Model file for the job. Use its own axes, mm. Face numbers are marked on the shaded views. A direction names the side the tool comes from. Coordinates: 2 decimals unless noted, no trailing zeros. Write each loop counter-clockwise with the first axis right and the second up, starting at its lowest first coordinate (ties: lowest second). Pieces come first, ordered by that corner, then holes.
Q1. Which spindle directions (+Z, -Z, +X, -X, +Y, -Y) get a long thin tool onto all of the face, cutting with end or side? Do the marked faces 1, 2 and 3. Say none if no direction does.
Q2. Drill centre lines: probe 1 along Y at (x, z) = (3.75, -9); probe 2 along X at (y, z) = (17.25, 0); probe 3 along Z at (x, y) = (-11.25, 7). Where is each one in solid material? Low to high.
Q3. Band-saw the part on C-C, the plane z = 1. State how many separate pieces and enclosed holes the cut face has, plus the area to 3 significant figures.
Q4. Band-saw the part on B-B, the plane x = -1.5. Write the cut outline in (y, z).
Q5. Band-saw the part on D-D, the plane y = 9. Write the cut outline in (x, z), plus the area to 3 significant figures.
Q6. Pin check, flat tips, straight feed: P1, Ø5.5, axis at y = 5, z = 1, coming from the -X side; P2, Ø10, axis at x = -4, z = -4, coming from the -Y side; P3, Ø12, axis at x = 1.5, z = -2, coming from the -Y side; P4, Ø3, axis at y = 13.5, z = 6.5, coming from the +X side. Stop position of each tip, or through.
Q7. Pull direction Z, two halves, no side cores. Call the marked faces 4, 5 and 6: released by +Z, released by -Z, zero draft, split by the parting line, or undercut.
Q8. Band-saw the part on A-A, the plane y = 39. Write the cut outline in (x, z), plus the area to 3 significant figures.
from build123d import *

# Parameters (mm, degrees)
SKETCH1_R               = 12.7
BOSS_EXTRUDE1_DEPTH     = 45.3136
CUT_EXTRUDE1_START      = -11.43
CUT_EXTRUDE1_DEPTH      = 11.43
CUT_EXTRUDE2_DEPTH      = 11.43
CUT_EXTRUDE3_DEPTH      = 52.259289353
CUT_EXTRUDE3_DEPTH_BACK = 52.259289353
SKETCH4_R               = 3.175
SKETCH5_R               = 2.54
CUT_EXTRUDE4_DEPTH      = 39.349424517
BOSS_EXTRUDE2_REACH     = 53.259
BOSS_EXTRUDE3_DEPTH     = 1.27


with BuildPart() as part:
    # Sketch1 → Boss-Extrude1 (new body)
    with BuildSketch(Plane(origin=(0, 0, 0), x_dir=(1, 0, 0), z_dir=(0, 1, 0))):
        with Locations(Location((0, 0, 0), (0, 0, 90))):
            Circle(SKETCH1_R)
    extrude(amount=BOSS_EXTRUDE1_DEPTH)

    # Sketch2 → Cut-Extrude1 (cut)
    with BuildSketch(Plane(origin=(0, 45.3136, 0), x_dir=(1, 0, 0), z_dir=(0, 1, 0)).offset(CUT_EXTRUDE1_START)):
        with BuildLine():
            Line((7.62, 10.16), (7.62, -10.16))
            ThreePointArc((7.62, -10.16), (0, -12.7), (-7.62, -10.16))
            Line((-7.62, -10.16), (-7.62, 10.16))
            ThreePointArc((-7.62, 10.16), (0, 12.7), (7.62, 10.16))
        make_face()
    extrude(amount=CUT_EXTRUDE1_DEPTH, mode=Mode.SUBTRACT)

    # Sketch3 → Cut-Extrude2 (cut)
    with BuildSketch(Plane.XZ):
        with BuildLine():
            Line((-7.62, 10.16), (-7.62, -10.16))
            ThreePointArc((-7.62, -10.16), (0, -12.7), (7.62, -10.16))
            Line((7.62, -10.16), (7.62, 10.16))
            ThreePointArc((7.62, 10.16), (0, 12.7), (-7.62, 10.16))
        make_face()
    extrude(amount=-CUT_EXTRUDE2_DEPTH, mode=Mode.SUBTRACT)

    # Sketch4 → Cut-Extrude3 (cut, two sides: drawn at the far end of the back side and taken through both)
    with BuildSketch(Plane(origin=(-7.62, 0, 0), x_dir=(0, 0, -1), z_dir=(1, 0, 0)).offset(-CUT_EXTRUDE3_DEPTH_BACK)):
        with Locations(Location((0, 40.2336, 0), (0, 0, 270))):
            Circle(SKETCH4_R)
        with Locations(Location((0, 5.08, 0), (0, 0, 270))):
            Circle(SKETCH4_R)
        with BuildLine():
            Line((0, 45.3136), (-10.16, 45.3136))
            Line((-10.16, 45.3136), (-10.16, 33.8836))
            Line((-10.16, 33.8836), (-4.264917923, 42.993468677))
            ThreePointArc((-4.264917923, 42.993468677), (-2.427577715, 44.696028312), (0, 45.3136))
        make_face()
        with BuildLine():
            Line((-10.16, 11.43), (-10.16, 0))
            Line((-10.16, 0), (0, 0))
            ThreePointArc((0, 0), (-2.427577715, 0.617571688), (-4.264917923, 2.320131323))
            Line((-4.264917923, 2.320131323), (-10.16, 11.43))
        make_face()
    extrude(amount=CUT_EXTRUDE3_DEPTH + CUT_EXTRUDE3_DEPTH_BACK, mode=Mode.SUBTRACT)

    # Sketch5 → Cut-Extrude4 (cut, through all)
    with BuildSketch(Plane(origin=(0, 33.8836, 0), x_dir=(1, 0, 0), z_dir=(0, 1, 0))):
        with Locations(Location((0, 0, 0), (0, 0, 270))):
            Circle(SKETCH5_R)
    extrude(amount=-CUT_EXTRUDE4_DEPTH, mode=Mode.SUBTRACT)

    # Boss-Extrude2: up to this face of the body (flat: up to its plane)
    boss_extrude2_end = Plane(part.part.faces().sort_by_distance((7.62, 34.116741009, 0))[0])
    # Sketch6 → Boss-Extrude2 (add, up to the picked face)
    with BuildSketch(Plane(origin=(-7.62, 0, 0), x_dir=(0, 0, -1), z_dir=(1, 0, 0)), mode=Mode.PRIVATE) as boss_extrude2_sk1:
        Polygon((2.54, 33.8836), (10.16, 33.8836), (10.16, 35.1536), (7.62, 35.1536), align=None)
    boss_extrude2_tool1 = split(extrude(boss_extrude2_sk1.sketch, amount=BOSS_EXTRUDE2_REACH, mode=Mode.PRIVATE), bisect_by=boss_extrude2_end, keep=Keep.BOTH, mode=Mode.PRIVATE)
    add(boss_extrude2_tool1.solids().sort_by(Axis((-7.62, 34.412767, -7.408333), (1, 0, 0)))[0])

    # Sketch7 → Boss-Extrude3 (add)
    with BuildSketch(Plane(origin=(0, 33.8836, 0), x_dir=(1, 0, 0), z_dir=(0, 1, 0))):
        with BuildLine():
            Line((-7.62, 10.16), (7.62, 10.16))
            ThreePointArc((7.62, 10.16), (0, 12.7), (-7.62, 10.16))
        make_face()
    extrude(amount=BOSS_EXTRUDE3_DEPTH)


solid = part.part
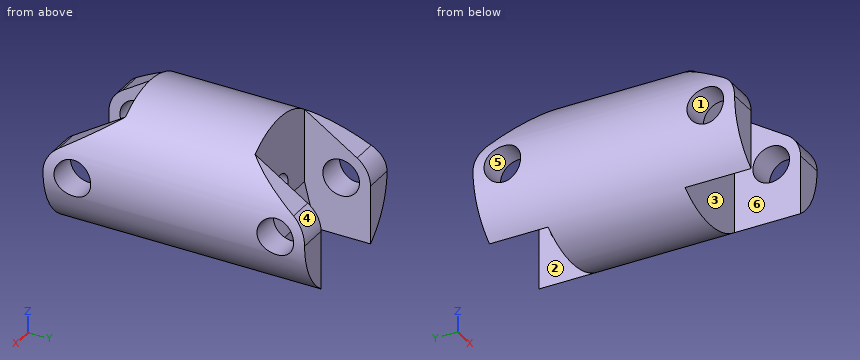
Answer sheet:
1. face 1: +X, -X
1. face 2: +Z, +Y
1. face 3: +Z, -Z, -Y
2. probe 1: y = 11.43 to 35.15
2. probe 2: x = -12.7 to -2.54, 2.54 to 12.7
2. probe 3: z = -5.89 to -2.53, 2.53 to 5.89
3. separate pieces: 6
3. enclosed holes: 0
3. area: 571 mm2
4. outline: (11.43, -12.61) - (35.15, -12.61) - (35.15, -7.62) - (33.88, -2.54) - (33.88, -2.05) - (11.43, -2.05) - close; (11.43, 2.05) - (33.88, 2.05) - (33.88, 12.61) - (11.43, 12.61) - close
5. outline: (-9.36, 8.59) arc R12.7 ccw to (-7.62, -10.16) - (-7.62, 8.59) - close; (7.62, -10.16) arc R12.7 ccw to (9.36, 8.59) - (7.62, 8.59) - close
5. area: 141 mm2
6. P1: stops at x = -12.61
6. P2: stops at y = 0
6. P3: stops at y = 11.43
6. P4: stops at x = 11.67
7. face 4: released by +Z
7. face 5: undercut
7. face 6: zero draft
8. outline: (-12.36, -2.93) arc R12.7 ccw to (-7.62, -10.16) - (-7.62, -2.93) - close; (-12.36, 2.93) - (-7.62, 2.93) - (-7.62, 6.85) - (-10.69, 6.85) arc R12.7 ccw to start; (7.62, -10.16) arc R12.7 ccw to (12.36, -2.93) - (7.62, -2.93) - close; (7.62, 2.93) - (12.36, 2.93) arc R12.7 ccw to (10.69, 6.85) - (7.62, 6.85) - close
8. area: 74.8 mm2
